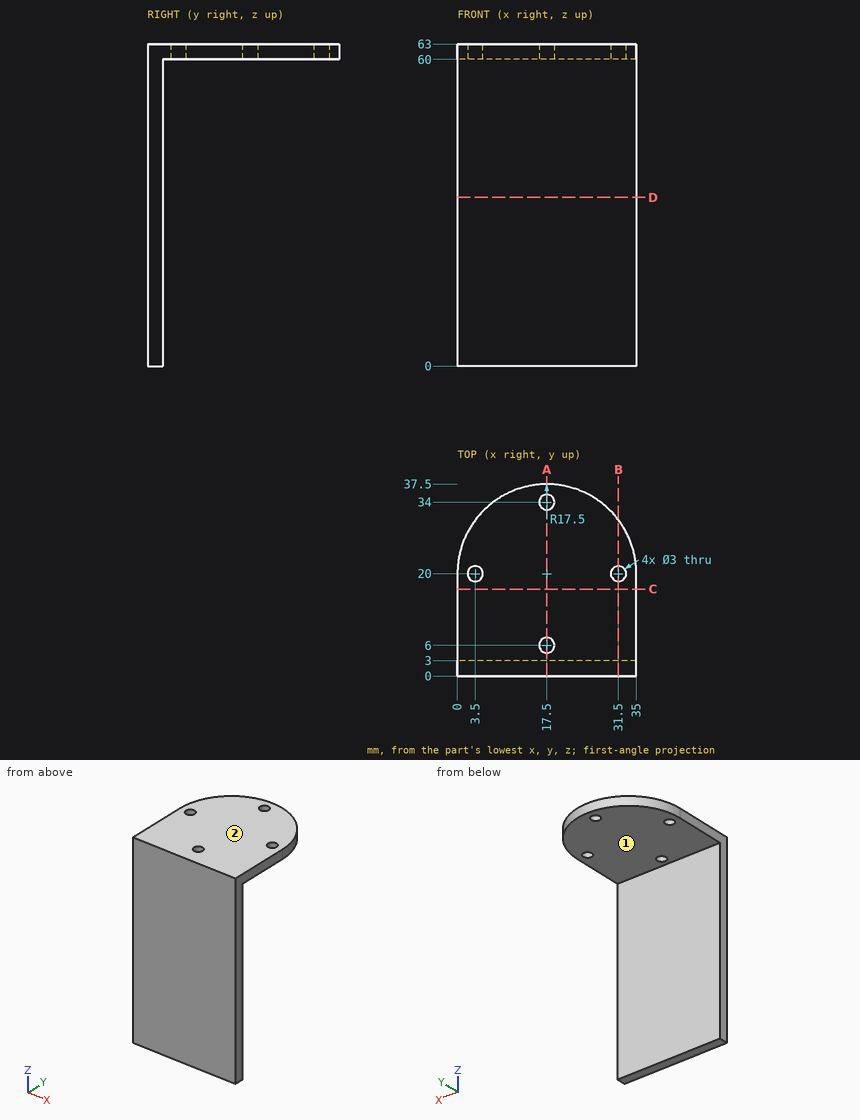
For this review, use the dimensioned drawing (mm, ordinates from the lowest corner) and the shaded views. A direction names the side the tool comes from. Give positions to 0.01 mm unless a question says otherwise; leave off trailing zeros. Loops run counter-clockwise (first coordinate to the right, second up) from the corner with the lowest first, then second, coordinate; pieces in that order, holes last.
Item 1: Insertion check: pin 1 (3.5 mm diameter, centred on x = 17.5, y = 34, fed in from +Z); pin 2 (2.5 mm diameter, centred on x = 3.5, y = 20, fed in from -Z); pin 3 (1.5 mm diameter, centred on x = 29, z = 48.5, fed in from +Y); pin 4 (2 mm diameter, centred on x = 20, y = 9, fed in from -Z). Each pin has a flat end and moves straight along its axis. Give the tip position at first contact, or say it passes through.
Item 2: Take a section at A-A, the plane x = 17.5. State the section outline as (y, z) points, and give its area (4 significant figures).
Item 3: Take a section at B-B, the plane x = 31.5. State the section outline as (y, z) points, and give its area (4 significant figures).
Item 4: For line 1 along Y through (x, z) = (17.5, 61.05); line 2 along Z through (x, y) = (4.5, 8.5); line 3 along Y through (x, z) = (31, 61), list the stretches that pass through material, from the lowest coordinate up.
Item 5: Tool access review of the marked faces 1 and 2: name each direction out of +Z, -Z, +X, -X, +Y, -Y from which nothing blocks a thin tool from reaching the whole face with its end or side.
Item 6: Take a section at C-C, the plane y = 17. State the section outline as (x, z) points.
Item 7: Take a section at D-D, the plane z = 33. State the section outline as (x, y) points, and give its area (3 significant figures).
Calculated:
1. pin 1: stops at z = 63
1. pin 2: passes through
1. pin 3: stops at y = 3
1. pin 4: stops at z = 60
2. outline: (0, 0) - (3, 0) - (3, 60) - (4.5, 60) - (4.5, 63) - (0, 63) - close; (7.5, 60) - (32.5, 60) - (32.5, 63) - (7.5, 63) - close; (35.5, 60) - (37.5, 60) - (37.5, 63) - (35.5, 63) - close
2. area: 274.5 mm2
3. outline: (0, 0) - (3, 0) - (3, 60) - (18.5, 60) - (18.5, 63) - (0, 63) - close; (21.5, 60) - (30.5, 60) - (30.5, 63) - (21.5, 63) - close
3. area: 262.5 mm2
4. line 1: y = 0 to 4.5, 7.5 to 32.5, 35.5 to 37.5
4. line 2: z = 60 to 63
4. line 3: y = 0 to 18.59, 21.41 to 31.14
5. face 1: -Z, +X, -X, +Y
5. face 2: +Z, +X, -X, +Y, -Y
6. outline: (0, 60) - (35, 60) - (35, 63) - (0, 63) - close
7. outline: (0, 0) - (35, 0) - (35, 3) - (0, 3) - close
7. area: 105 mm2
